Geometry check sheet. Reference: the model listing, model coordinates, mm. Round coordinates to 2 decimals unless told otherwise and drop trailing zeros. Write each loop counter-clockwise with the first axis right and the second up, starting at its lowest first coordinate (ties: lowest second). Pieces come first, ordered by that corner, then holes. Notation, with made-up numbers: (34.5, 0.5) -> (71.5, 0.5) arc R22 cw to (71.5, 17.5) -> close; hole circle Ø3 at (63, 36.5). An arc over 180 degrees is marked (long way). Return JSON: item names as keys, results as strings. Group by question number.
from build123d import *

# Parameters (mm, degrees)
BOSS_EXTRUDE1_DEPTH = 6.35
SKETCH2_R           = 1.5
CUT_EXTRUDE1_DEPTH  = 212
SKETCH3_R           = 1.5
CUT_EXTRUDE2_DEPTH  = 212
SKETCH4_R           = 1.375
CUT_EXTRUDE3_DEPTH  = 212
SKETCH5_R           = 1.5
CUT_EXTRUDE4_DEPTH  = 212
SKETCH6_R           = 2
CUT_EXTRUDE5_DEPTH  = 212


with BuildPart() as part:
    # Sketch1 → Boss-Extrude1 (new body)
    with BuildSketch(Plane(origin=(0, 0, 0), x_dir=(1, 0, 0), z_dir=(0, 1, 0))):
        with BuildLine():
            Line((-246.189194392, 203.762814663), (-108.786796564, 66.360416836))
            ThreePointArc((-108.786796564, 66.360416836), (-102.283614025, 56.627716371), (-100, 45.1472134))
            Line((-100, 45.1472134), (-100, -45.1472134))
            ThreePointArc((-100, -45.1472134), (-102.283614025, -56.627716371), (-108.786796564, -66.360416836))
            Line((-108.786796564, -66.360416836), (-246.189194392, -203.762814663))
            ThreePointArc((-246.189194392, -203.762814663), (-246.225197781, -246.201202305), (-203.786796564, -246.213203436))
            Line((-203.786796564, -246.213203436), (-66.360389693, -108.786796564))
            ThreePointArc((-66.360389693, -108.786796564), (-56.627689229, -102.283614025), (-45.147186258, -100))
            Line((-45.147186258, -100), (45.147186258, -100))
            ThreePointArc((45.147186258, -100), (56.627689229, -102.283614025), (66.360389693, -108.786796564))
            Line((66.360389693, -108.786796564), (203.786796564, -246.213203436))
            ThreePointArc((203.786796564, -246.213203436), (246.225197781, -246.201202305), (246.189194392, -203.762814663))
            Line((246.189194392, -203.762814663), (108.786796564, -66.360416836))
            ThreePointArc((108.786796564, -66.360416836), (102.283614025, -56.627716371), (100, -45.1472134))
            Line((100, -45.1472134), (100, 45.1472134))
            ThreePointArc((100, 45.1472134), (102.283614025, 56.627716371), (108.786796564, 66.360416836))
            Line((108.786796564, 66.360416836), (246.189194392, 203.762814663))
            ThreePointArc((246.189194392, 203.762814663), (246.225197781, 246.201202305), (203.786796564, 246.213203436))
            Line((203.786796564, 246.213203436), (66.360389693, 108.786796564))
            ThreePointArc((66.360389693, 108.786796564), (56.627689229, 102.283614025), (45.147186258, 100))
            Line((45.147186258, 100), (-45.147186258, 100))
            ThreePointArc((-45.147186258, 100), (-56.627689229, 102.283614025), (-66.360389693, 108.786796564))
            Line((-66.360389693, 108.786796564), (-203.786796564, 246.213203436))
            ThreePointArc((-203.786796564, 246.213203436), (-246.225197781, 246.201202305), (-246.189194392, 203.762814663))
        make_face()
    extrude(amount=BOSS_EXTRUDE1_DEPTH)

    # Sketch2 → Cut-Extrude1 (cut)
    with BuildSketch(Plane(origin=(0, 6.35, 0), x_dir=(1, 0, 0), z_dir=(0, 1, 0))):
        with Locations((-225, 241.5)):
            Circle(SKETCH2_R)
        with Locations((-208.5, 225)):
            Circle(SKETCH2_R)
        with Locations((-225, 208.5)):
            Circle(SKETCH2_R)
        with Locations((-241.5, 225)):
            Circle(SKETCH2_R)
        with Locations((241.5, 225)):
            Circle(SKETCH2_R)
        with Locations((225, 241.5)):
            Circle(SKETCH2_R)
        with Locations((208.5, 225)):
            Circle(SKETCH2_R)
        with Locations((225, 208.5)):
            Circle(SKETCH2_R)
        with Locations((225, -241.5)):
            Circle(SKETCH2_R)
        with Locations((241.5, -225)):
            Circle(SKETCH2_R)
        with Locations((225, -208.5)):
            Circle(SKETCH2_R)
        with Locations((208.5, -225)):
            Circle(SKETCH2_R)
        with Locations((-241.5, -225)):
            Circle(SKETCH2_R)
        with Locations((-225, -241.5)):
            Circle(SKETCH2_R)
        with Locations((-208.5, -225)):
            Circle(SKETCH2_R)
        with Locations((-225, -208.5)):
            Circle(SKETCH2_R)
    extrude(amount=-CUT_EXTRUDE1_DEPTH, mode=Mode.SUBTRACT)

    # Sketch3 → Cut-Extrude2 (cut)
    with BuildSketch(Plane(origin=(0, 6.35, 0), x_dir=(1, 0, 0), z_dir=(0, 1, 0))):
        with Locations((-7.62, 10.795)):
            Circle(SKETCH3_R)
        with Locations((-7.62, -10.795)):
            Circle(SKETCH3_R)
        with Locations((7.62, -10.795)):
            Circle(SKETCH3_R)
        with Locations((7.62, 10.795)):
            Circle(SKETCH3_R)
    extrude(amount=-CUT_EXTRUDE2_DEPTH, mode=Mode.SUBTRACT)

    # Sketch4 → Cut-Extrude3 (cut)
    with BuildSketch(Plane(origin=(0, 6.35, 0), x_dir=(1, 0, 0), z_dir=(0, 1, 0))):
        with Locations((-24.5, 21)):
            Circle(SKETCH4_R)
        with Locations((24.5, 21)):
            Circle(SKETCH4_R)
        with Locations((24.5, 79)):
            Circle(SKETCH4_R)
        with Locations((-24.5, 79)):
            Circle(SKETCH4_R)
    extrude(amount=-CUT_EXTRUDE3_DEPTH, mode=Mode.SUBTRACT)

    # Sketch5 → Cut-Extrude4 (cut)
    with BuildSketch(Plane(origin=(0, 6.35, 0), x_dir=(1, 0, 0), z_dir=(0, 1, 0))):
        with Locations((24.15, -30)):
            Circle(SKETCH5_R)
        with Locations((-24.15, -30)):
            Circle(SKETCH5_R)
        with Locations((-16.141801743, -81.683254161)):
            Circle(SKETCH5_R)
        with Locations((11.857903914, -81.554867605)):
            Circle(SKETCH5_R)
    extrude(amount=-CUT_EXTRUDE4_DEPTH, mode=Mode.SUBTRACT)

    # Sketch6 → Cut-Extrude5 (cut)
    with BuildSketch(Plane(origin=(0, 6.35, 0), x_dir=(1, 0, 0), z_dir=(0, 1, 0))):
        with Locations((75, 75)):
            Circle(SKETCH6_R)
        with Locations((65, 65)):
            Circle(SKETCH6_R)
        with Locations((50, 50)):
            Circle(SKETCH6_R)
        with Locations((50, -50)):
            Circle(SKETCH6_R)
        with Locations((65, -65)):
            Circle(SKETCH6_R)
        with Locations((75, -75)):
            Circle(SKETCH6_R)
        with Locations((-50, -50)):
            Circle(SKETCH6_R)
        with Locations((-65, -65)):
            Circle(SKETCH6_R)
        with Locations((-75, -75)):
            Circle(SKETCH6_R)
        with Locations((-50, 50)):
            Circle(SKETCH6_R)
        with Locations((-65, 65)):
            Circle(SKETCH6_R)
        with Locations((-75, 75)):
            Circle(SKETCH6_R)
    extrude(amount=-CUT_EXTRUDE5_DEPTH, mode=Mode.SUBTRACT)


solid = part.part
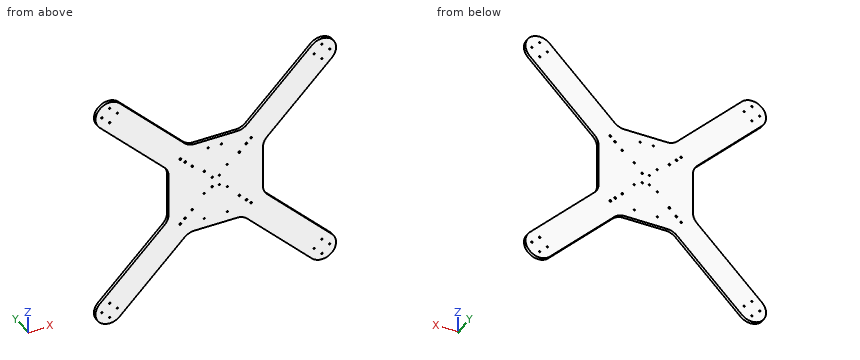
1) Sectioned sample at D-D on y = 2.75. State how many separate pieces and enclosed holes the cut face has, and give its area (3 significant figures).
2) Material ranges on probe 1 along Z at (x, y) = (65, 4); probe 2 along X at (y, z) = (2, -75), recorded low to high. Write a range as [from, to].
3) Go/stop test with flat-tipped pins: P1, Ø2.5, axis at x = -75, z = 75, coming from the -Y side; P2, Ø1, axis at x = 69.5, y = 4, coming from the +Z side. Record where each tip stops, or that it passes through.
4) Sectioned sample at C-C on z = 2.5. Enter the section's corners in (x, y), and give its area (3 significant figures).
5) Sectioned sample at B-B on x = 155. Enter the section's corners in (y, z).
6) Sectioned sample at A-A on z = 155.5. Enter the section's corners in (x, y).
Evaluation:
{
 "1": {"separate pieces": "1", "enclosed holes": "40", "area": "91,500 mm2"},
 "2": {"probe 1": "z = [-107.51, -67], [-63, 63], [67, 107.51]", "probe 2": "x = [-117.43, -77], [-73, 73], [77, 117.43]"},
 "3": {"P1": "passes through", "P2": "stops at z = 112.43"},
 "4": {"outline": "(-100, 0) -> (100, 0) -> (100, 6.35) -> (-100, 6.35) -> close", "area": "1,270 mm2"},
 "5": {"outline": "(0, -197.43) -> (6.35, -197.43) -> (6.35, -112.57) -> (0, -112.57) -> close; (0, 112.57) -> (6.35, 112.57) -> (6.35, 197.43) -> (0, 197.43) -> close"},
 "6": {"outline": "(-197.93, 0) -> (-113.07, 0) -> (-113.07, 6.35) -> (-197.93, 6.35) -> close; (113.07, 0) -> (197.93, 0) -> (197.93, 6.35) -> (113.07, 6.35) -> close"}
}
